Could you check a few things on this model? Use its own coordinates, in mm. Face numbers are marked on the shaded views. Give positions to 0.01 mm unless a question says otherwise; leave off trailing zeros. Order: outer loops, then holes, each group sorted by start corner. A loop starts at its lowest first (then second) coordinate and runs counter-clockwise, first axis right, second up. Notation, with made-up numbers: (65, 14) - (85, 14) arc R18 ccw to (85, 45) - close; hole circle Ø9 at (20.25, 34.5). An arc over 180 degrees is marked (long way). One line per question, with ' | ' between items. Start each with the question number.
1. Imagine slicing it at A-A (x = 0). Please give me the cut outline in (y, z).
2. For P1, Ø4, axis at y = 5, z = 3, coming from the -X side; P2, Ø1.5, axis at y = 5, z = -1, coming from the +X side; P3, Ø4, axis at x = 2, y = 6.5, coming from the -Z side, each with a flat end and sliding along its axis, tell me the tip position at first contact or that it passes through.
3. If we mould it in two halves opening along Y, with no side actions, what happens to the marked faces 1, 2, 3 and 4? For each: released by +Y, released by -Y, zero draft, split by the parting line, or undercut.
4. I need wall thicknesses on probe 1 along X at (y, z) = (14.5, 0); probe 2 along X at (y, z) = (8.75, 0); probe 3 along Y at (x, z) = (-2, 1.25). Which ranges of each line are inside material? Lowest first, please. Write a range as from..to.
5. Imagine slicing it at C-C (x = 4.5). Please give me the cut outline in (y, z).
6. Imagine slicing it at D-D (y = 12.25). Please give me the cut outline in (x, z).
7. Imagine slicing it at B-B (z = 4). Please give me the cut outline in (x, y).
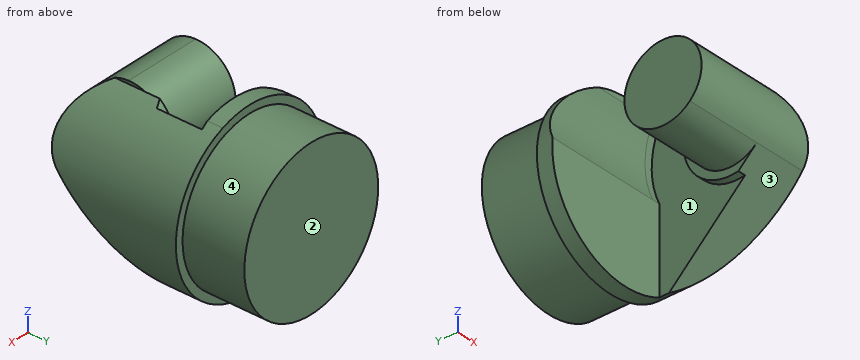
```python
from build123d import *

# Parameters (mm, degrees)
SKETCH1_W               = 11
SKETCH1_H               = 11
BOSS_EXTRUDE1_DEPTH     = 15
SKETCH2_R               = 11.526525906
SKETCH2_R_2             = 5
CUT_EXTRUDE1_DEPTH      = 4
SKETCH3_R               = 9.335544837
SKETCH3_R_2             = 5.5
CUT_EXTRUDE2_DEPTH      = 1
CUT_EXTRUDE4_DEPTH      = 20.397164741
CUT_EXTRUDE5_DEPTH      = 7.5
SKETCH7_R               = 4.206819523
CUT_EXTRUDE6_DEPTH      = 2.5
SKETCH8_R               = 8.743774997
CUT_EXTRUDE7_DEPTH      = 12.521718622
SKETCH9_R               = 5.5
SKETCH9_R_2             = 2.5
CUT_EXTRUDE8_DEPTH      = 5
CUT_EXTRUDE8_DEPTH_BACK = 5
CUT_EXTRUDE9_DEPTH      = 0.5


with BuildPart() as part:
    # Sketch1 → Boss-Extrude1 (new body)
    with BuildSketch(Plane(origin=(0, 0, 0), x_dir=(1, 0, 0), z_dir=(0, 1, 0))):
        Rectangle(SKETCH1_W, SKETCH1_H)
    extrude(amount=BOSS_EXTRUDE1_DEPTH)

    # Sketch2 → Cut-Extrude1 (cut)
    with BuildSketch(Plane(origin=(0, 15, 0), x_dir=(1, 0, 0), z_dir=(0, 1, 0))):
        Circle(SKETCH2_R)
        with Locations(Location((0, 0, 0), (0, 0, 270))):
            Circle(SKETCH2_R_2, mode=Mode.SUBTRACT)
    extrude(amount=-CUT_EXTRUDE1_DEPTH, mode=Mode.SUBTRACT)

    # Sketch3 → Cut-Extrude2 (cut)
    with BuildSketch(Plane(origin=(0, 11, 0), x_dir=(1, 0, 0), z_dir=(0, 1, 0))):
        Circle(SKETCH3_R)
        with Locations(Location((0, 0, 0), (0, 0, 270))):
            Circle(SKETCH3_R_2, mode=Mode.SUBTRACT)
    extrude(amount=-CUT_EXTRUDE2_DEPTH, mode=Mode.SUBTRACT)

    # Sketch4 → Cut-Extrude4 (cut, through all)
    with BuildSketch(Plane.ZY.offset(5.5)):
        with BuildLine():
            Line((1.028660662, 3.260538449), (-5.5, 10))
            Line((-5.5, 10), (-9.452355575, 12.560239237))
            Line((-9.452355575, 12.560239237), (-9.996263861, -3.051690792))
            Line((-9.996263861, -3.051690792), (13.077304092, -2.572417867))
            Line((13.077304092, -2.572417867), (11.793537329, 10))
            Line((11.793537329, 10), (5.5, 10))
            Line((5.5, 10), (5.32277104, 4.912954629))
            ThreePointArc((5.32277104, 4.912954629), (3.722129922, 2.666788079), (1.028660662, 3.260538449))
        make_face()
    extrude(amount=-CUT_EXTRUDE4_DEPTH, mode=Mode.SUBTRACT)

    # Sketch6 → Cut-Extrude5 (cut)
    with BuildSketch(Plane.ZY.offset(5.5)):
        with BuildLine():
            Line((5.32277104, 4.912954629), (5.5, 10))
            Line((5.5, 10), (-5.5, 10))
            Line((-5.5, 10), (1.028660662, 3.260538449))
            ThreePointArc((1.028660662, 3.260538449), (1.926443835, 7.333211921), (5.32277104, 4.912954629))
        make_face()
    extrude(amount=-CUT_EXTRUDE5_DEPTH, mode=Mode.SUBTRACT)

    # Sketch7 → Cut-Extrude6 (cut)
    with BuildSketch(Plane.ZY.offset(5.5)):
        with Locations((2.824286879, 5)):
            Circle(SKETCH7_R)
    extrude(amount=-CUT_EXTRUDE6_DEPTH, mode=Mode.SUBTRACT)

    # Sketch8 → Cut-Extrude7 (cut, through all)
    with BuildSketch(Plane(origin=(0, 11, 0), x_dir=(1, 0, 0), z_dir=(0, 1, 0))):
        Circle(SKETCH8_R)
        with BuildLine():
            Line((0, -5.5), (2, -5.5))
            Line((2, -5.5), (2, -5.123475383))
            ThreePointArc((2, -5.123475383), (0.790050421, 5.442960622), (-3.374127459, -4.343416154))
            Line((-3.374127459, -4.343416154), (-3.374127459, -5.5))
            Line((-3.374127459, -5.5), (0, -5.5))
        make_face(mode=Mode.SUBTRACT)
    extrude(amount=-CUT_EXTRUDE7_DEPTH, mode=Mode.SUBTRACT)

    # Sketch9 → Cut-Extrude8 (cut, two sides)
    with BuildSketch(Plane.ZY.offset(3)) as cut_extrude8_sk:
        with Locations((2.824286879, 5)):
            Circle(SKETCH9_R)
        with Locations((2.824286879, 5)):
            Circle(SKETCH9_R_2, mode=Mode.SUBTRACT)
    extrude(amount=CUT_EXTRUDE8_DEPTH, mode=Mode.SUBTRACT)
    extrude(cut_extrude8_sk.sketch, amount=-CUT_EXTRUDE8_DEPTH_BACK, mode=Mode.SUBTRACT)

    # Sketch10 → Cut-Extrude9 (cut)
    with BuildSketch(Plane.ZY.offset(-2)):
        with BuildLine():
            ThreePointArc((-0.125167599, 4.451622134), (1.544554545, 7.71335312), (5.123475383, 6.927104621))
            Line((5.123475383, 6.927104621), (5.123475383, 9.996371906))
            ThreePointArc((5.123475383, 9.996371906), (5.119525771, 9.998187514), (5.115574726, 10))
            ThreePointArc((5.115574726, 10), (2.824286879, 10.5), (0.532999031, 10))
            Line((0.532999031, 10), (-5.123475383, 10))
            Line((-5.123475383, 10), (-5.123475383, 9.611317955))
            Line((-5.123475383, 9.611317955), (-2.379973921, 6.779232849))
            Line((-2.379973921, 6.779232849), (-0.125167599, 4.451622134))
        make_face()
    extrude(amount=-CUT_EXTRUDE9_DEPTH, mode=Mode.SUBTRACT)


solid = part.part
```
Results found:
1) outline: circle Ø5 at (5, 2.82); (10, -5.5) - (11, -5.5) - (11, -5) - (15, -5) - (15, 5) - (11, 5) - (11, 5.5) - (10, 5.5) - (10, 5.12) arc R5.5 cw to (10, 0.53) - close
2) P1: stops at x = -3 | P2: stops at x = 5.49 | P3: stops at z = -3.99
3) face 1: undercut | face 2: released by +Y | face 3: released by -Y | face 4: zero draft
4) probe 1: x = -5..5 | probe 2: x = 2.5..5.5 | probe 3: y = 3.06..6.94, 10.27..15
5) outline: (2.52, 3.16) arc R2.5 ccw to (3.26, 1.03) - (7.59, -3.16) - (11, -3.16) - (11, -2.18) - (15, -2.18) - (15, 2.18) - (11, 2.18) - (11, 3.16) - close
6) outline: circle Ø10 at (0, 0)
7) outline: (-3.77, 10.37) - (2.5, 10.37) - (2.5, 7.76) - (2, 7.76) - (2, 7.21) - (-3, 7.21) - (-3, 2.79) - (3.77, 2.79) - (3.77, 11) - (3, 11) - (3, 15) - (-3, 15) - (-3, 11) - (-3.77, 11) - close
